Geometry check sheet. Reference: the model listing, model coordinates, mm. A direction names the side the tool comes from. Coordinates: 2 decimals unless noted, no trailing zeros. Write each loop counter-clockwise with the first axis right and the second up, starting at its lowest first coordinate (ties: lowest second). Pieces come first, ordered by that corner, then holes.
from build123d import *

# Parameters (mm, degrees)
SKETCH1_W           = 7
SKETCH1_H           = 6
BOSS_EXTRUDE1_DEPTH = 5.05
SKETCH3_W           = 0.68
SKETCH3_H           = 0.27
BOSS_EXTRUDE2_DEPTH = 4.3
SKETCH4_W           = 0.4
SKETCH4_H           = 5.8
BOSS_EXTRUDE3_DEPTH = 6.9
SKETCH6_W           = 6.67
SKETCH6_H           = 1.45
CUT_EXTRUDE1_DEPTH  = 13.06410896
CUT_EXTRUDE2_REACH  = 10.686
SKETCH7_W           = 1.5
SKETCH7_H           = 0.53
BOSS_EXTRUDE5_START = -3.6
SKETCH9_R           = 0.5
BOSS_EXTRUDE5_DEPTH = 4
BOSS_EXTRUDE6_DEPTH = 0.4
BOSS_EXTRUDE4_START = -1
BOSS_EXTRUDE4_DEPTH = 1


with BuildPart() as part:
    # Sketch1 → Boss-Extrude1 (new body)
    with BuildSketch(Plane(origin=(0, 0, 0), x_dir=(1, 0, 0), z_dir=(0, 1, 0))):
        Rectangle(SKETCH1_W, SKETCH1_H)
    extrude(amount=BOSS_EXTRUDE1_DEPTH)

    # Sketch3 → Boss-Extrude2 (add)
    with BuildSketch(Plane.XY.offset(3)):
        with Locations((-2.22, 2.595)):
            Rectangle(SKETCH3_W, SKETCH3_H)
        with Locations((2.22, 2.595)):
            Rectangle(SKETCH3_W, SKETCH3_H)
    extrude(amount=BOSS_EXTRUDE2_DEPTH)

    # Sketch4 → Boss-Extrude3 (add)
    with BuildSketch(Plane(origin=(0, 0, -3), x_dir=(-1, 0, 0), z_dir=(0, 0, -1))):
        with Locations((-3.535, 2.15)):
            Rectangle(SKETCH4_W, SKETCH4_H)
        with Locations((3.535, 2.15)):
            Rectangle(SKETCH4_W, SKETCH4_H)
    extrude(amount=-BOSS_EXTRUDE3_DEPTH)

    # Sketch6 → Cut-Extrude1 (cut, through all)
    with BuildSketch(Plane(origin=(0, 0, -3), x_dir=(-1, 0, 0), z_dir=(0, 0, -1))):
        with Locations((0, 0.725)):
            Rectangle(SKETCH6_W, SKETCH6_H)
    extrude(amount=-CUT_EXTRUDE1_DEPTH, mode=Mode.SUBTRACT)

    # Sketch7 → Cut-Extrude2 (cut, up to next)
    with BuildSketch(Plane.XY.offset(3), mode=Mode.PRIVATE) as cut_extrude2_sk1:
        with Locations((0, 1.715)):
            Rectangle(SKETCH7_W, SKETCH7_H)
    cut_extrude2_tool1 = extrude(cut_extrude2_sk1.sketch, amount=-CUT_EXTRUDE2_REACH, mode=Mode.PRIVATE) & part.part
    add(cut_extrude2_tool1.solids().sort_by_distance((0, 1.715, 3))[0], mode=Mode.SUBTRACT)

    # Sketch9 → Boss-Extrude5 (add)
    with BuildSketch(Plane(origin=(0, 5.05, 0), x_dir=(1, 0, 0), z_dir=(0, 1, 0)).offset(BOSS_EXTRUDE5_START)):
        with Locations(Location((-3.095, 2.36, 0), (0, 0, 90))):
            Circle(SKETCH9_R)
        with Locations(Location((-3.095, -2.36, 0), (0, 0, 90))):
            Circle(SKETCH9_R)
        with Locations(Location((3.095, 2.36, 0), (0, 0, 90))):
            Circle(SKETCH9_R)
        with Locations(Location((3.095, -2.36, 0), (0, 0, 90))):
            Circle(SKETCH9_R)
    extrude(amount=BOSS_EXTRUDE5_DEPTH)

    # Sketch2 → Revolve1 (revolve)
    with BuildSketch(Plane.XY):
        Polygon((0, 5.05), (0, 10.95), (1.5, 10.95), (1.75, 5.05), align=None)
    revolve(axis=Axis((0, 5.05, 0), (0, 1, 0)))

    # Sketch10 → Boss-Extrude6 (add)
    with BuildSketch(Plane.ZY.offset(3.735)):
        Polygon((3.9, -0.75), (3.9, -1.35), (1.1, -1.35), (-3, -0.75), align=None)
    boss_extrude6 = extrude(amount=-BOSS_EXTRUDE6_DEPTH)

    # Sketch8 → Boss-Extrude4 (add)
    with BuildSketch(Plane.XZ.offset(1.35).offset(BOSS_EXTRUDE4_START)):
        Polygon((-3.735, 3.9), (-3.735, 4.3), (-4.335, 5.18), (-3.721940695, 7.52), (-3.335, 7.41862496), (-3.901894327, 5.254833117), (-3.335, 4.423388104), (-3.335, 3.9), align=None)
    boss_extrude4 = extrude(amount=-BOSS_EXTRUDE4_DEPTH)

    # Mirror1: Boss-Extrude6, Boss-Extrude4 across plane
    add(boss_extrude6.mirror(Plane(origin=(0, 0, 0), x_dir=(0, 0, 1), z_dir=(1, 0, 0))))
    add(boss_extrude4.mirror(Plane(origin=(0, 0, 0), x_dir=(0, 0, 1), z_dir=(1, 0, 0))))


solid = part.part
1. Sectioned sample at B-B, the plane z = 2.36. Record the boundary of the cut face in (x, y) (3 decimals), and give its area (3 significant figures).
Computed values:
outline: (-3.735, -1.35) - (-3.335, -1.35) - (-3.335, 1.45) - (-0.75, 1.45) - (-0.75, 1.98) - (0.75, 1.98) - (0.75, 1.45) - (3.335, 1.45) - (3.335, -1.35) - (3.735, -1.35) - (3.735, 5.05) - (3.595, 5.05) - (3.595, 5.45) - (2.595, 5.45) - (2.595, 5.05) - (-2.595, 5.05) - (-2.595, 5.45) - (-3.595, 5.45) - (-3.595, 5.05) - (-3.735, 5.05) - close
area: 29.1 mm2
2. Sectioned sample at C-C, the plane x = 0. Record the boundary of the cut face in (y, z), and give its area (3 significant figures).
Computed values:
outline: (1.98, -3) - (5.05, -3) - (5.05, -1.75) - (10.95, -1.5) - (10.95, 1.5) - (5.05, 1.75) - (5.05, 3) - (1.98, 3) - close
area: 37.6 mm2
3. Gauge pin test, flat ends, axial feed: pin 1 Ø3 at (x, y) = (1, 2) entering from +Z; pin 2 Ø0.5 at (x, z) = (4, 5.5) entering from -Y; pin 3 Ø3 at (x, y) = (-0.5, 7.5) entering from -Z. Record the tip position at first contact, or that the pin passes through.
Computed values:
pin 1: stops at z = 7.3
pin 2: stops at y = -0.35
pin 3: stops at z = -1.71
4. Draft check along Z on faces 4 (the cylindrical face through (3.29, 5.25, -2.82)), 5 (the flat face through (4.033, 0.143, 6.334)), 6 (the flat face through (4.03, 0.14, 4.73)). Enter one of: released by +Z, released by -Z, zero draft, split by the parting line, or undercut.
Computed values:
face 4: undercut
face 5: released by +Z
face 6: released by -Z
5. Thickness scan on line 1 along X through (y, z) = (0, -1.5) (3 decimals); line 2 along Z through (x, y) = (2.5, 2.5); line 3 along X through (y, z) = (1.75, 1) (3 decimals). Record the ranges inside material, lowest first.
Computed values:
line 1: x = -3.735 to -3.335, 3.335 to 3.735
line 2: z = -3 to 7.3
line 3: x = -3.735 to -0.75, 0.75 to 3.735
6. Sectioned sample at D-D, the plane z = 5.75. Record the boundary of the cut face in (x, y).
Computed values:
outline: (-4.19, -0.35) - (-3.77, -0.35) - (-3.77, 0.65) - (-4.19, 0.65) - close; (-2.56, 2.46) - (-1.88, 2.46) - (-1.88, 2.73) - (-2.56, 2.73) - close; (1.88, 2.46) - (2.56, 2.46) - (2.56, 2.73) - (1.88, 2.73) - close; (3.77, -0.35) - (4.19, -0.35) - (4.19, 0.65) - (3.77, 0.65) - close
7. Access from +Z, -Z, +X, -X, +Y, -Y to the whole of each face (thin tool, end or side, straight path). Record for faces 1 (the flat face through (-3.335, 0, 1)), 2 (the cylindrical face through (3.29, 5.25, 1.9)), 3 (the flat face through (-3.735, 2, 1)).
Computed values:
face 1: +Z, -Y
face 2: +Y
face 3: -Z, -X, +Y, -Y
8. Sectioned sample at A-A, the plane y = -0.5. Record the boundary of the cut face in (x, z) (3 decimals), and give its area (3 significant figures).
Computed values:
outline: (-3.735, -3) - (-3.335, -3) - (-3.335, 3.9) - (-3.735, 3.9) - close; (3.335, -3) - (3.735, -3) - (3.735, 3.9) - (3.335, 3.9) - close
area: 5.52 mm2
